Read the model definition and answer for the solid it produces. Units are mm, in the model's axes. A direction names the side the tool comes from. Coordinates: 2 decimals unless noted, no trailing zeros. Loops run counter-clockwise (first coordinate to the right, second up) from the corner with the lowest first, then second, coordinate; pieces in that order, holes last.
Q1. Section C-C (x = -12.5) is taken. Give the vertices of the cut face in (y, z).
Q2. A flat-ended cylindrical pin translates along its axis: P1, Ø1.5, axis at x = -1, z = 4.5, coming from the +Y side. Find the tip coordinate at first contact, or state that the pin passes through.
Q3. Which of the six approach directions +Z, -Z, +X, -X, +Y, -Y give full straight-line access (tool end or side, diameter ignored) to faces 1 (the face through (7.73, 2.46, 1.5)), 2 (the face through (0, -5, -12.5))?
Q4. The mould has two halves that part along X. Classify faces 3 (the face through (-12, 5, 0)), 4 (the face through (0, 0, 0)), 5 (the face through (-25, -5, 0)), 6 (the face through (25, -5, 0)): pulls with the +X half, pulls with the -X half, needs draft (parallel to the pull), parting line crosses it, or undercut.
Q5. Section A-A (z = 0) is taken. Give the vertices of the cut face in (x, y), then the cut area to 3 significant figures.
Q6. Section D-D (z = -2.75) is taken. Give the vertices of the cut face in (x, y), then the cut area to 3 significant figures.
Q7. Section B-B (y = 0.5) is taken. Give the vertices of the cut face in (x, z), then the cut area to 3 significant figures.
Q8. Straight lines are drawn through the part: line 1 (Y direction, x = 7.5, z = -10.5); line 2 (X direction, y = 2.5, z = 1); line 3 (Z direction, x = -9, y = 3.5). For each, find the intervals that lie inside material, in ascending order.
from build123d import *

# Parameters (mm, degrees)
F0_W     = 50
F0_H     = 25
F1_DEPTH = 10
F2_R     = 5
F3_DEPTH = 5


with BuildPart() as f1:
    # F0 (on Front) → F1 (new body)
    with BuildSketch(Plane.XZ):
        Rectangle(F0_W, F0_H)
    extrude(amount=F1_DEPTH)

    # F2 (on face) → F3 (join)
    with BuildSketch(Plane(origin=(0, 0, 0), x_dir=(-1, 0, 0), z_dir=(0, 1, 0))):
        with Locations((-12.5, 0)):
            Circle(F2_R)
        with Locations((12.5, 0)):
            Circle(F2_R)
    extrude(amount=F3_DEPTH)


solid = f1.part
Numbers:
1. outline: (-10, -12.5) - (0, -12.5) - (0, -5) - (5, -5) - (5, 5) - (0, 5) - (0, 12.5) - (-10, 12.5) - close
2. P1: stops at y = 0
3. face 1: +Y
3. face 2: -Z, +X, -X, +Y, -Y
4. face 3: needs draft
4. face 4: undercut
4. face 5: pulls with the -X half
4. face 6: pulls with the +X half
5. outline: (-25, -10) - (25, -10) - (25, 0) - (17.5, 0) - (17.5, 5) - (7.5, 5) - (7.5, 0) - (-7.5, 0) - (-7.5, 5) - (-17.5, 5) - (-17.5, 0) - (-25, 0) - close
5. area: 600 mm2
6. outline: (-25, -10) - (25, -10) - (25, 0) - (16.68, 0) - (16.68, 5) - (8.32, 5) - (8.32, 0) - (-8.32, 0) - (-8.32, 5) - (-16.68, 5) - (-16.68, 0) - (-25, 0) - close
6. area: 584 mm2
7. outline: circle Ø10 at (-12.5, 0); circle Ø10 at (12.5, 0)
7. area: 157 mm2
8. line 1: y = -10 to 0
8. line 2: x = -17.4 to -7.6, 7.6 to 17.4
8. line 3: z = -3.57 to 3.57
